```python
from build123d import *

# Parameters (mm, degrees)
BOSS_EXTRUDE1_DEPTH = 60.324999999999996
SKETCH2_R           = 6.349999999999996
SKETCH2_R_2         = 3.174999999999997
SKETCH2_R_3         = 6.350000000000003
BOSS_EXTRUDE2_DEPTH = 23.8125
FILLET1_R           = 6.35
SHELL1_START        = 3.175
SHELL1_DEPTH        = 53.975
SHELL1_START_2      = 9.525
SHELL1_2_DEPTH      = 41.275


# Read off the part's stored shape, not the designer's step: Shell1
with BuildPart() as part:
    # Sketch1 → Boss-Extrude1 (new body)
    with BuildSketch(Plane(origin=(0, 0, 0), x_dir=(0, 0, -1), z_dir=(1, 0, 0))):
        with BuildLine():
            Line((95.25, -46.808484128263686), (56.59005614988863, -64.27972260468273))
            ThreePointArc((56.59005614988863, -64.27972260468273), (55.235212183230196, -64.71688198003586), (53.81702677554687, -64.84122281357011))
            Line((53.81702677554687, -64.84122281357011), (0.1579732244523257, -63.50589713864123))
            ThreePointArc((0.1579732244523257, -63.50589713864123), (-7.8219e-13, -63.5039318313911), (-0.15797322445388826, -63.50589713864123))
            Line((-0.15797322445388826, -63.50589713864123), (-53.817026775546886, -64.84122281357013))
            ThreePointArc((-53.817026775546886, -64.84122281357013), (-57.54105224821803, -63.747307586818266), (-59.93275370705406, -60.69038423543624))
            Line((-59.93275370705406, -60.69038423543624), (-66.28275370705404, -43.47219611461599))
            Line((-66.28275370705404, -43.47219611461599), (-65.6463, -71.1931881208203))
            Line((-65.6463, -71.1931881208203), (95.25, -71.19318812082028))
            Line((95.25, -71.19318812082028), (95.25, -46.808484128263686))
        make_face()
    extrude(amount=BOSS_EXTRUDE1_DEPTH)

    # Sketch2 → Boss-Extrude2 (add, symmetric)
    # profile 1 of 2: a face of its own
    with BuildSketch(Plane(origin=(30.162499999999998, 0, 0), x_dir=(0, 0, -1), z_dir=(1, 0, 0))):
        with Locations((-53.975, -58.49318812082027)):
            Circle(SKETCH2_R)
        with Locations((-53.975, -58.49318812082027)):
            Circle(SKETCH2_R_2, mode=Mode.SUBTRACT)
    # profile 2 of 2: a face of its own
    with BuildSketch(Plane(origin=(30.162499999999998, 0, 0), x_dir=(0, 0, -1), z_dir=(1, 0, 0))):
        with Locations((53.97499999999999, -58.49318812082027)):
            Circle(SKETCH2_R_3)
        with Locations((53.97499999999999, -58.49318812082027)):
            Circle(SKETCH2_R_2, mode=Mode.SUBTRACT)
    extrude(amount=BOSS_EXTRUDE2_DEPTH, both=True)

    # Fillet1
    fillet1_edges = [part.edges().sort_by_distance(p)[0] for p in [
        (30.162499999999998, -60.69038423543624, 59.93275370705406),
        (30.162499999999998, -64.84122281357013, 53.817026775546886),
        (30.162499999999998, -64.27972260468273, -56.59005614988863),
        (30.162499999999998, -64.84122281357011, -53.81702677554687),
    ]]
    fillet(fillet1_edges, radius=FILLET1_R)

    # Shell1 outline → Shell1 (cut)
    with BuildSketch(Plane.YZ.offset(SHELL1_START)):
        with BuildLine():
            Line((-66.679914485, 0.078986612), (-68.01524016, 53.738040163))
            ThreePointArc((-68.01524016, 53.738040163), (-66.547807009, 59.059165573), (-62.375448989, 62.672912138))
            Line((-62.375448989, 62.672912138), (-71.193188121, 62.470463295))
            Line((-71.193188121, 62.470463295), (-71.193188121, -92.075))
            Line((-71.193188121, -92.075), (-51.727499707, -92.075))
            Line((-51.727499707, -92.075), (-67.172989847, -57.897584225))
            ThreePointArc((-67.172989847, -57.897584225), (-67.82872891, -55.865318275), (-68.01524016, -53.738040163))
            Line((-68.01524016, -53.738040163), (-66.679914485, -0.078986612))
            ThreePointArc((-66.679914485, -0.078986612), (-66.678931831, 0), (-66.679914485, 0.078986612))
        make_face()
    extrude(amount=SHELL1_DEPTH, mode=Mode.SUBTRACT)

    # Shell1 2 outline → Shell1 2 (cut)
    with BuildSketch(Plane.YZ.offset(SHELL1_START_2)):
        with BuildLine():
            ThreePointArc((-67.699293711, 41.041970778), (-66.500168266, 45.910832805), (-62.99442515, 49.496008461))
            ThreePointArc((-62.99442515, 49.496008461), (-63.747307587, 57.541052248), (-55.99280194, 59.811999995))
            ThreePointArc((-55.99280194, 59.811999995), (-55.617794314, 61.369720704), (-54.986992393, 62.842545699))
            Line((-54.986992393, 62.842545699), (-62.375448989, 62.672912138))
            ThreePointArc((-62.375448989, 62.672912138), (-66.547807009, 59.059165573), (-68.01524016, 53.738040163))
            Line((-68.01524016, 53.738040163), (-67.699293711, 41.041970778))
        make_face()
        with BuildLine():
            ThreePointArc((-62.99442515, -49.496008461), (-66.500168266, -45.910832805), (-67.699293711, -41.041970778))
            Line((-67.699293711, -41.041970778), (-68.01524016, -53.738040163))
            ThreePointArc((-68.01524016, -53.738040163), (-67.82872891, -55.865318275), (-67.172989847, -57.897584225))
            Line((-67.172989847, -57.897584225), (-61.942877547, -69.470653193))
            ThreePointArc((-61.942877547, -69.470653193), (-62.732304839, -64.518832939), (-60.897427959, -59.85225538))
            ThreePointArc((-60.897427959, -59.85225538), (-64.71688198, -55.235212183), (-62.99442515, -49.496008461))
        make_face()
    extrude(amount=SHELL1_2_DEPTH, mode=Mode.SUBTRACT)


solid = part.part
```
CAD build for the part. Positions are in the model's coordinates, mm. A direction names the side the tool comes from. Give positions to 0.01 mm unless a question says otherwise; leave off trailing zeros. Order: outer loops, then holes, each group sorted by start corner. A loop starts at its lowest first (then second) coordinate and runs counter-clockwise, first axis right, second up.
(1) Mould opens along Y. For faces 1 (the cylindrical face through (29.874, -55.625, 61.348)), 2 (the flat face through (59, -71.193, 9)), 3 (the flat face through (6.35, -55, 55)) say: released by +Y, released by -Y, zero draft, split by the parting line, or undercut.
(2) Saw through at A-A, the plane x = 48. State how many separate pieces and enclosed holes the cut face has, then the cut area to 3 significant figures.
(3) Flat gauge pins, fed straight in: pin 1 (6 mm diameter, centred on y = -57.5, z = -45, fed in from +X) (3 decimals); pin 2 (12 mm diameter, centred on x = 25.5, y = -55.5, fed in from +Z); pin 3 (1.5 mm diameter, centred on x = 52, y = -49.5, fed in from +Z); pin 4 (4 mm diameter, centred on y = -58.49, z = 53.98, fed in from -X). Where does each tip first touch, or does it go through?
(4) Tool access for faces 4 (the flat face through (53.975, -55, 55)), 5 (the flat face through (6.35, -62, -54)): list every direction of +Z, -Z, +X, -X, +Y, -Y with a clear straight run to the whole face (end or side of a thin tool).
(5) Saw through at B-B, the plane z = -82. Give the cut face in (x, y) (3 decimals).
(6) Saw through at C-C, the plane z = -10. Give the cut face in (x, y) (3 decimals).
(7) Drill centre lines: L1, parallel to X at y = -68.75, z = 50 (3 decimals); L2, parallel to Z at x = 10.5, y = -60.5 (3 decimals); L3, parallel to Z at x = 16.5, y = -52 (3 decimals). Where is each one in solid material? Low to high.
Results found:
1. face 1: undercut
1. face 2: released by -Y
1. face 3: zero draft
2. separate pieces: 1
2. enclosed holes: 2
2. area: 784 mm2
3. pin 1: stops at x = 53.975
3. pin 2: stops at z = 66.14
3. pin 3: stops at z = 66.16
3. pin 4: passes through
4. face 4: +X, +Y
4. face 5: -X, +Y
5. outline: (0, -71.193) - (3.175, -71.193) - (3.175, -56.281) - (57.15, -56.281) - (57.15, -71.193) - (60.325, -71.193) - (60.325, -52.796) - (0, -52.796) - close
6. outline: (0, -71.193) - (3.175, -71.193) - (3.175, -66.927) - (57.15, -66.927) - (57.15, -71.193) - (60.325, -71.193) - (60.325, -63.751) - (0, -63.751) - close
7. L1: x = 0 to 3.175, 57.15 to 60.325
7. L2: z = -95.25 to -92.075, -72.663 to -56.435, -51.515 to -47.189, 47.189 to 51.515, 56.435 to 60, 62.716 to 65.892
7. L3: z = -95.25 to -92.075, -91.472 to -83.762, 61.674 to 66.087
